Autodesk Inventor part; units mm, degrees
ref_plane "YZ Plane" through (0, 0, 0) normal (1, 0, 0) x (0, 1, 0)
ref_plane "XZ Plane" through (0, 0, 0) normal (0, 1, 0) x (-1, 0, 0)
ref_plane "XY Plane" through (0, 0, 0) normal (0, 0, 1) x (1, 0, 0)
sketch "Esboço1" plane through (0, 0, 0) normal (0, 0, 1) x (1, 0, 0)
  line L0 (0, 0) -> (143, 0)
  line L1 (0, 14.5) -> (16.5, 14.5)
  line L2 (45.5, 14.5) -> (45.5, 6)
  line L3 (143, 0) -> (113, 0)
  line L4 (45.5, 14.5) -> (113, 7.75)
  arc A0 (143, 18.4741) -> (118.8287, 22.9497) centre (130.5, 18.4741) ccw
  line L5 (113, 7.75) -> (118.8287, 22.9497)
  line L6 (0, -14.5) -> (2, -14.5)
  line L7 (2, -14.5) -> (2, -11.5)
  line L8 (18.9914, 6) -> (45.5, 6)
  line L9 (16.5, 14.5) -> (18.9914, 6)
  line L10 (27, -14.5) -> (25, -14.5)
  line L11 (25, -14.5) -> (25, -11.5)
  line L12 (2, -11.5) -> (25, -11.5)
  line L13 (143, -5.6516) -> (129.0406, -6.7164)
  arc A1 (127.3817, -11.2647) -> (129.06, -10.2586) centre (129.8143, -13.4198) ccw
  circle A2 centre (129.8143, -13.4198) radius 1
  arc A3 (126.0492, -6.9446) -> (127.3817, -11.2647) centre (132.7451, -7.2449) ccw
  arc A4 (129.0406, -6.7164) -> (129.06, -10.2586) centre (132.2697, -8.4698) ccw
  line L14 (27, -14.5) -> (126.0492, -6.9446)
  line L15 (129.0406, -6.7164) -> (143, -5.6516)
  line L16 (-14.5, 0) -> (-0.5, 0)
  line L17 (-0.5, 0) -> (-0.5, -3)
  line L18 (-0.5, -3) -> (-14.1863, -3)
  arc A5 (0, 14.5) -> (-14.5, 0) centre (0, 0) ccw
  arc A6 (-14.1863, -3) -> (0, -14.5) centre (0, 0) ccw
  line L19 (113, 7.75) -> (124.9404, 6.556)
  line L20 (143, 10.75) -> (129, 10.75)
  line L21 (129, 10.75) -> (129, 7.75)
  line L22 (129, 7.75) -> (143, 7.75)
  line L23 (143, -5.6516) -> (143, 7.75)
  line L24 (143, 10.75) -> (143, 18.4741)
  dimension "d1" = 143
  dimension "d5" = 29
  dimension "d6" = 8.5
  dimension "d23" = 2
  dimension "d24" = 3
  dimension "d67" = 6.5
  dimension "d68" = 2
  dimension "d85" = 14
  dimension "d86" = 3
  dimension "d87" = 12
  dimension "d91" = 14
extrude "Extrusão1" add sketch "Esboço1" along normal blind 3
sketch "Esboço2" plane through (0, 0, 3) normal (0, 0, 1) x (1, 0, 0)
  line L0 (113, 7.75) -> (45.5, 14.5)
  line L1 (45.5, 14.5) -> (140.0285, 5.0471)
  arc A0 (140.0458, 4.0541) -> (140.0285, 5.0471) centre (139.9788, 4.5496) ccw
  line L2 (18.9914, 6) -> (16.5, 14.5)
  line L3 (25, -11.5) -> (140.0458, 4.0541)
  line L4 (45.5, 6) -> (18.9914, 6)
  line L5 (18.9914, 6) -> (45.5, 6)
  line L6 (45.5, 6) -> (45.5, 14.5)
  line L7 (9, -11.5) -> (9, -14.5)
  line L8 (9, -14.5) -> (12, -14.5)
  line L9 (12, -14.5) -> (12, -11.5)
  line L10 (6, -11.5) -> (9, -11.5)
  line L11 (18, -11.5) -> (18, -14.5)
  line L12 (18, -14.5) -> (15, -14.5)
  line L13 (15, -14.5) -> (15, -11.5)
  line L14 (12, -11.5) -> (15, -11.5)
  line L15 (18, -11.5) -> (25, -11.5)
  line L16 (-12.5, 0) -> (-12.5, 0.25)
  arc A1 (-12.3593, 0.4749) -> (-12.5, 0.25) centre (-12.25, 0.25) ccw
  line L17 (16.5, 14.5) -> (-12.3593, 0.4749)
  line L18 (-12.5, -3) -> (-12.5, -3.25)
  arc A2 (-12.5, -3.25) -> (-12.3501, -3.4791) centre (-12.25, -3.25) ccw
  line L19 (6, -11.5) -> (-12.3501, -3.4791)
  line L20 (-12.5, 0) -> (-0.5, 0)
  line L21 (-0.5, 0) -> (-0.5, -3)
  line L22 (-0.5, -3) -> (-12.5, -3)
  point P0 (0, 0)
  point P1 (113, 7.75)
  dimension "d22" = 95
  dimension "d45" = 3
  dimension "d46" = 3
  dimension "d48" = 3
  dimension "d49" = 3
  dimension "d60" = 3
  dimension "d82" = 12
extrude "Extrusão2" add sketch "Esboço2" along normal blind 3
sketch "Esboço3" plane through (0, 0, 0) normal (0, 0, -1) x (-1, 0, 0)
  arc A0 (-140.0285, 5.0471) -> (-140.0458, 4.0541) centre (-139.9788, 4.5496) ccw
  arc A1 (-140.0285, 5.0471) -> (-140.0458, 4.0541) centre (-139.9788, 4.5496) ccw
  line L0 (-25, -11.5) -> (-140.0458, 4.0541)
  line L1 (-45.5, 14.5) -> (-45.5, 6)
  line L2 (-45.5, 14.5) -> (-45.5, 6)
  line L3 (-45.5, 6) -> (-18.9914, 6)
  line L4 (-25, -11.5) -> (-18, -11.5)
  line L5 (-18.9914, 6) -> (-16.5, 14.5)
  arc A2 (12.5, 0.25) -> (12.3593, 0.4749) centre (12.25, 0.25) ccw
  arc A3 (12.5, 0.25) -> (12.3593, 0.4749) centre (12.25, 0.25) ccw
  arc A4 (12.3501, -3.4791) -> (12.5, -3.25) centre (12.25, -3.25) ccw
  arc A5 (12.3501, -3.4791) -> (12.5, -3.25) centre (12.25, -3.25) ccw
  line L6 (-15, -14.5) -> (-18, -14.5)
  line L7 (-18, -11.5) -> (-18, -14.5)
  line L8 (-18, -14.5) -> (-15, -14.5)
  line L9 (-15, -14.5) -> (-15, -11.5)
  line L10 (-12, -14.5) -> (-12, -11.5)
  line L11 (-15, -11.5) -> (-12, -11.5)
  line L12 (-12, -11.5) -> (-12, -14.5)
  line L13 (-9, -11.5) -> (-9, -14.5)
  line L14 (-12, -14.5) -> (-9, -14.5)
  line L15 (-9, -14.5) -> (-9, -11.5)
  line L16 (12.3501, -3.4791) -> (-6, -11.5)
  line L17 (-9, -11.5) -> (-6, -11.5)
  line L18 (-6, -11.5) -> (12.3501, -3.4791)
  line L19 (-16.5, 14.5) -> (12.3593, 0.4749)
  line L20 (-16.5, 14.5) -> (12.3593, 0.4749)
  line L21 (-140.0285, 5.0471) -> (-45.5, 14.5)
  line L22 (-45.5, 14.5) -> (-140.0285, 5.0471)
  line L23 (12.5, -3.25) -> (12.5, -3)
  line L24 (12.5, 0) -> (12.5, 0.25)
  line L25 (12.5, 0) -> (0.5, 0)
  line L26 (0.5, 0) -> (0.5, -3)
  line L27 (0.5, -3) -> (12.5, -3)
  point P0 (12.3501, -3.4791)
  point P1 (12.3593, 0.4749)
  point P2 (12.3593, 0.4749)
  point P3 (12.5, 0.25)
  point P4 (12.5, -3.25)
  point P5 (12.3501, -3.4791)
extrude "Extrusão3" add sketch "Esboço3" along normal blind 3
properties part number "CORPO"
Could you check a few things on this model? Use its own coordinates, in mm. A direction names the side the tool comes from. Give positions to 0.01 mm unless a question says otherwise; leave off trailing zeros. Loops run counter-clockwise (first coordinate to the right, second up) from the corner with the lowest first, then second, coordinate; pieces in that order, holes last. Notation, with made-up numbers: M 28,35 L 39,35 A22 ccw 39,52 Z; hole C 20,-20 d9. An arc over 180 degrees is marked long. Answer as a JSON object with one key per item and string values.
Q1. For P1, Ø0.9, axis at y = -12.5, z = -1.5, coming from the +X side; P2, Ø2.5, axis at x = 10.5, z = -1.5, coming from the -Y side; P3, Ø1, axis at x = 22, z = 1, coming from the -Y side, each with a flat end and sliding along its axis, tell me the tip position at first contact or that it passes through.
Values found:
{"P1": "stops at x = 18", "P2": "stops at y = -14.5", "P3": "stops at y = -11.5"}
Q2. Suppose I cut it at C-C, the plane y = -1.5. List the corners of the cut face in (x, z) for me.
Values found:
{"outline": "M -0.5,-3 L 98.96,-3 L 98.96,0 L 143,0 L 143,3 L 98.96,3 L 98.96,6 L -0.5,6 Z"}
Q3. Suppose I cut it at A-A, the plane z = 1.5. List the corners of the cut face in (x, y) for me.
Values found:
{"outline": "M -14.5,0 L -0.5,0 L -0.5,-3 L -14.19,-3 A14.5 ccw 0,-14.5 L 2,-14.5 L 2,-11.5 L 25,-11.5 L 25,-14.5 L 27,-14.5 L 126.05,-6.94 A6.7 ccw 127.38,-11.26 A3.25 ccw long 129.06,-10.26 A3.67 cw 129.04,-6.72 L 143,-5.65 L 143,7.75 L 129,7.75 L 129,10.75 L 143,10.75 L 143,18.47 A12.5 ccw 118.83,22.95 L 113,7.75 L 45.5,14.5 L 45.5,6 L 18.99,6 L 16.5,14.5 L 0,14.5 A14.5 ccw Z; hole C 129.81,-13.42 d2"}
Q4. If I drill on probe 1 along X at (y, z) = (-14, -0.5); probe 2 along Z at (x, y) = (128, 18.5); probe 3 along Y at (x, z) = (23.5, 2.75), over which ranges is the centre line in solid material (lowest first)? Write a range as [from, to].
Values found:
{"probe 1": "x = [9, 12], [15, 18]", "probe 2": "z = [0, 3]", "probe 3": "y = [-11.5, 6]"}
Q5. For faces 4 (the flat face through (136, 7.75, 1)), 5 (the flat face through (18, -13, 4)), 6 (the flat face through (8, 14.5, 1)), which set-ups out of +Z, -Z, +X, -X, +Y, -Y let a thin tool reach every point of the face, with its end or its side?
Values found:
{"face 4": "+Z, -Z, +X", "face 5": "+Z, -Z, +X, -Y", "face 6": "+Z, -Z, -X, +Y"}
Q6. If we mould it in two halves opening along Z, with no side actions, what happens to faces 1 (the flat face through (-3, 9, 3)), 2 (the flat face through (-0.5, -1, 2)), 3 (the flat face through (10, -13, 3))? For each: pulls with the +Z half, pulls with the -Z half, needs draft (parallel to the pull), parting line crosses it, or undercut.
Values found:
{"face 1": "pulls with the +Z half", "face 2": "needs draft", "face 3": "undercut"}
